Geometry check sheet. Reference: the model listing, model coordinates, mm. Give positions to 0.01 mm unless a question says otherwise; leave off trailing zeros. Write each loop counter-clockwise with the first axis right and the second up, starting at its lowest first coordinate (ties: lowest second). Pieces come first, ordered by that corner, then holes.
(1) Cross-section at C-C (x = 8.5). Record the boundary of the cut face in (y, z), and give its area (3 significant figures).
(2) Cross-section at B-B (y = -1.5). Record the boundary of the cut face in (x, z).
(3) Depth check by flat-ended pin: P1, Ø0.6, axis at y = -76.5, z = 1, coming from the -X side; P2, Ø1, axis at x = -7, z = 0.5, coming from the +Y side; P3, Ø0.6, axis at x = 42, z = 1.5, coming from the +Y side; P4, Ø2.5, axis at x = 0, y = 13.5, coming from the +Z side. Enter the tip coordinate at first touch or a pass-through.
(4) Thickness scan on line 1 along X through (y, z) = (10, 1.35); line 2 along X through (y, z) = (-86.5, 1.6); line 3 along X through (y, z) = (26.5, 1.35). Record the ranges inside material, lowest first.
(5) Cross-section at D-D (z = 0.6). Count the separate pieces of the cut face and the enclosed holes in it, and give its area (3 significant figures).
(6) Cross-section at A-A (y = 13.5). Record the boundary of the cut face in (x, z).
```python
from build123d import *

# Parameters (mm, degrees)
SKETCH_3_R      = 2.2
SKETCH_3_R_2    = 1.5
EXTRUDE_1_DEPTH = 2


with BuildPart() as part:
    # 草图3 → 凸台-拉伸1 (new body)
    with BuildSketch(Plane.XY):
        with BuildLine():
            Line((-41.4, -74.890216685), (-41.4, -93.890216685))
            Line((-41.4, -93.890216685), (-30, -93.890216685))
            Line((-30, -93.890216685), (-30, -78.890216685))
            ThreePointArc((-30, -78.890216685), (-28.828427125, -76.061789561), (-26, -74.890216685))
            Line((-26, -74.890216685), (20.641271636, -74.890216685))
            ThreePointArc((20.641271636, -74.890216685), (23.469698761, -76.061789561), (24.641271636, -78.890216685))
            Line((24.641271636, -78.890216685), (24.641271636, -93.890216685))
            Line((24.641271636, -93.890216685), (24.641271636, -97.990216685))
            Line((24.641271636, -97.990216685), (24.641271636, -98.990216685))
            Line((24.641271636, -98.990216685), (43.741271636, -98.990216685))
            Line((43.741271636, -98.990216685), (45.741271636, -93.890216685))
            Line((45.741271636, -93.890216685), (45.741271636, 31.741152315))
            Line((45.741271636, 31.741152315), (45.230037269, 31.741152315))
            ThreePointArc((45.230037269, 31.741152315), (36.686440181, 34.468680322), (28.716551195, 30.356098435))
            ThreePointArc((28.716551195, 30.356098435), (27.478316584, 29.033500084), (26.179230338, 27.770619934))
            ThreePointArc((26.179230338, 27.770619934), (16.152230905, 17.515551518), (1.809761925, 17.542559084))
            ThreePointArc((1.809761925, 17.542559084), (0, 17.5), (-1.809761925, 17.542559084))
            ThreePointArc((-1.809761925, 17.542559084), (-15.928828372, 17.542283516), (-25.912710857, 27.525776288))
            ThreePointArc((-25.912710857, 27.525776288), (-27.223611076, 28.776388924), (-28.474223712, 30.087289143))
            ThreePointArc((-28.474223712, 30.087289143), (-36.482419799, 34.124770496), (-45, 31.317051182))
            Line((-45, 31.317051182), (-47, 31.317051182))
            Line((-47, 31.317051182), (-47, -74.890216685))
            Line((-47, -74.890216685), (-41.4, -74.890216685))
        make_face()
        with Locations((0, 13.5)):
            Circle(SKETCH_3_R, mode=Mode.SUBTRACT)
        with Locations((-30.052038202, 25.947961669)):
            Circle(SKETCH_3_R, mode=Mode.SUBTRACT)
        with Locations((30.199957913, 26.082571452)):
            Circle(SKETCH_3_R, mode=Mode.SUBTRACT)
        with Locations((42.5, -14.940216685)):
            Circle(SKETCH_3_R_2, mode=Mode.SUBTRACT)
        with Locations(Location((-42.5, -14.940216685, 0), (0, 0, 180))):
            Circle(SKETCH_3_R_2, mode=Mode.SUBTRACT)
        with Locations((42.5, -84.940216685)):
            Circle(SKETCH_3_R_2, mode=Mode.SUBTRACT)
        with BuildLine():
            Line((-43.6, -9.990216685), (-43.6, 25.009783315))
            ThreePointArc((-43.6, 25.009783315), (-42.5, 25.465418233), (-41.4, 25.009783315))
            Line((-41.4, 25.009783315), (-41.4, -9.990216685))
            ThreePointArc((-41.4, -9.990216685), (-42.5, -10.445851604), (-43.6, -9.990216685))
        make_face(mode=Mode.SUBTRACT)
        with BuildLine():
            Line((-41.4, -19.890216685), (-41.4, -25.190216685))
            Line((-41.4, -25.190216685), (-43.6, -25.190216685))
            Line((-43.6, -25.190216685), (-43.6, -19.890216685))
            ThreePointArc((-43.6, -19.890216685), (-42.5, -19.434581767), (-41.4, -19.890216685))
        make_face(mode=Mode.SUBTRACT)
        with BuildLine():
            Line((37.1, -93.890216685), (29.9, -93.890216685))
            Line((29.9, -93.890216685), (29.9, -96.090216685))
            Line((29.9, -96.090216685), (37.1, -96.090216685))
            ThreePointArc((37.1, -96.090216685), (37.555634919, -94.990216685), (37.1, -93.890216685))
        make_face(mode=Mode.SUBTRACT)
        with BuildLine():
            Line((43.6, -25.190216685), (43.6, -19.890216685))
            ThreePointArc((43.6, -19.890216685), (42.5, -19.434581767), (41.4, -19.890216685))
            Line((41.4, -19.890216685), (41.4, -25.190216685))
            Line((41.4, -25.190216685), (43.6, -25.190216685))
        make_face(mode=Mode.SUBTRACT)
        with BuildLine():
            Line((43.6, -95.190216685), (43.6, -89.890216685))
            ThreePointArc((43.6, -89.890216685), (42.5, -89.434581767), (41.4, -89.890216685))
            Line((41.4, -89.890216685), (41.4, -95.190216685))
            Line((41.4, -95.190216685), (43.6, -95.190216685))
        make_face(mode=Mode.SUBTRACT)
        with BuildLine():
            Line((41.4, -74.890216685), (41.4, -80.090216685))
            ThreePointArc((41.4, -80.090216685), (42.5, -80.545851604), (43.6, -80.090216685))
            Line((43.6, -80.090216685), (43.6, -74.890216685))
            Line((43.6, -74.890216685), (41.4, -74.890216685))
        make_face(mode=Mode.SUBTRACT)
        with BuildLine():
            Line((41.4, 25.009783315), (41.4, -9.990216685))
            ThreePointArc((41.4, -9.990216685), (42.5, -10.445851604), (43.6, -9.990216685))
            Line((43.6, -9.990216685), (43.6, 25.009783315))
            ThreePointArc((43.6, 25.009783315), (42.5, 25.465418233), (41.4, 25.009783315))
        make_face(mode=Mode.SUBTRACT)
        with BuildLine():
            Line((-21.830528741, -3.5), (26.741271636, -3.5))
            ThreePointArc((26.741271636, -3.5), (28.155485198, -4.085786438), (28.741271636, -5.5))
            Line((28.741271636, -5.5), (28.741271636, -50.70338646))
            ThreePointArc((28.741271636, -50.70338646), (27.539684971, -52.537108399), (25.378735489, -52.167454508))
            Line((25.378735489, -52.167454508), (-23.193064888, -6.964068047))
            ThreePointArc((-23.193064888, -6.964068047), (-23.691729441, -4.767926266), (-21.830528741, -3.5))
        make_face(mode=Mode.SUBTRACT)
        with BuildLine():
            Line((-26.637463853, -9.222762177), (21.934336524, -54.426148638))
            ThreePointArc((21.934336524, -54.426148638), (22.433001077, -56.62229042), (20.571800377, -57.890216685))
            Line((20.571800377, -57.890216685), (-28, -57.890216685))
            ThreePointArc((-28, -57.890216685), (-29.414213562, -57.304430248), (-30, -55.890216685))
            Line((-30, -55.890216685), (-30, -10.686830225))
            ThreePointArc((-30, -10.686830225), (-28.798413335, -8.853108286), (-26.637463853, -9.222762177))
        make_face(mode=Mode.SUBTRACT)
    extrude(amount=EXTRUDE_1_DEPTH)


solid = part.part
```
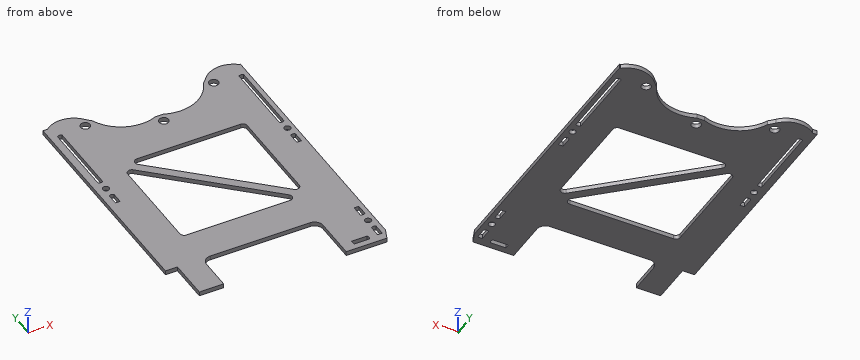
Reply:
1. outline: (-74.89, 0) - (-57.89, 0) - (-57.89, 2) - (-74.89, 2) - close; (-41.92, 0) - (-36.46, 0) - (-36.46, 2) - (-41.92, 2) - close; (-3.5, 0) - (16.09, 0) - (16.09, 2) - (-3.5, 2) - close
1. area: 84.1 mm2
2. outline: (-47, 0) - (-43.6, 0) - (-43.6, 2) - (-47, 2) - close; (-41.4, 0) - (41.4, 0) - (41.4, 2) - (-41.4, 2) - close; (43.6, 0) - (45.74, 0) - (45.74, 2) - (43.6, 2) - close
3. P1: stops at x = -41.4
3. P2: stops at y = 16.29
3. P3: stops at y = 33.79
3. P4: passes through
4. line 1: x = -47 to -43.6, -41.4 to 41.4, 43.6 to 45.74
4. line 2: x = -41.4 to -30, 24.64 to 45.74
4. line 3: x = -47 to -32.18, -27.92 to -25.45, 25.62 to 28.04, 32.36 to 45.74
5. separate pieces: 1
5. enclosed holes: 15
5. area: 6,810 mm2
6. outline: (-47, 0) - (-43.6, 0) - (-43.6, 2) - (-47, 2) - close; (-41.4, 0) - (-2.2, 0) - (-2.2, 2) - (-41.4, 2) - close; (2.2, 0) - (41.4, 0) - (41.4, 2) - (2.2, 2) - close; (43.6, 0) - (45.74, 0) - (45.74, 2) - (43.6, 2) - close
